Check sheet for the modelled part. Datum: model origin and axes. Units: mm. Face numbers are marked on the shaded views. A direction names the side the tool comes from. Round coordinates to 2 decimals unless told otherwise and drop trailing zeros. Loops run counter-clockwise (first coordinate to the right, second up) from the corner with the lowest first, then second, coordinate; pieces in that order, holes last. Notation, with made-up numbers: M 44,48 L 99,48 A19 cw 99,72 Z; hole C 15,-18 d11. An arc over 180 degrees is marked long. Write item = value, one per line. Start each with the question number.
(1) Cross-section at C-C on z = -1.25. Record the boundary of the cut face in (x, y), plus the area to 3 significant figures.
(2) Cross-section at B-B on x = -67.5. Record the boundary of the cut face in (y, z).
(3) Go/stop test with a flat-tipped pin: P1, Ø1, axis at x = -56, z = 2.5, coming from the -Y side. Record where the tip stops, or that it passes through.
(4) Scan lines: L1, parallel to Z at x = -48.5, y = 3; L2, parallel to Z at x = -27, y = -0.25; L3, parallel to X at y = -2, z = 0.75. Record each from-to range of solid material in increasing order. Write a range as from..to.
(5) Cross-section at A-A on y = 0. Record the boundary of the cut face in (x, z).
(6) Set-up check for the marked faces 1, 2 and 3: record each of +Z, -Z, +X, -X, +Y, -Y from which the full face is reachable in a straight line by a thin tool's end or side.
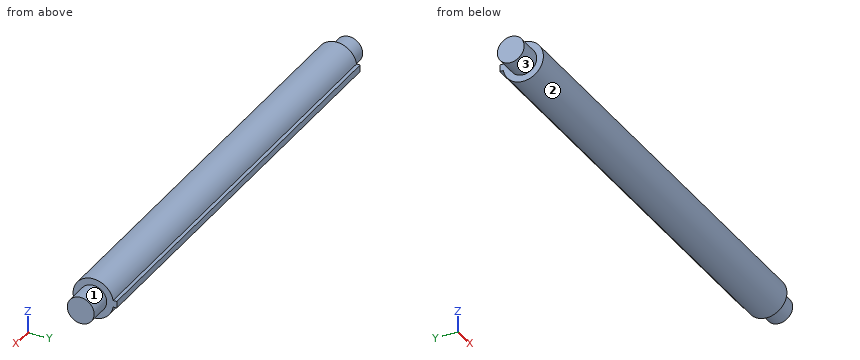
from build123d import *

# Parameters (mm, degrees)
SKETCH2_W           = 1
SKETCH2_H           = 1
BOSS_EXTRUDE1_DEPTH = 68


with BuildPart() as part:
    # Sketch1 → Revolve1 (revolve)
    with BuildSketch(Plane.XY):
        Polygon((0, 0), (-75, 0), (-75, 2), (-71.5, 2), (-71.5, 3), (-3.5, 3), (-3.5, 2), (0, 2), align=None)
    revolve(axis=Axis((0, 0, 0), (-1, 0, 0)))

    # Sketch2 → Boss-Extrude1 (add)
    with BuildSketch(Plane.ZY.offset(71.5)):
        with Locations((0, 3)):
            Rectangle(SKETCH2_W, SKETCH2_H)
    extrude(amount=-BOSS_EXTRUDE1_DEPTH)


solid = part.part
Result:
q1.outline = M -75,-1.56 L -71.5,-1.56 L -71.5,-2.73 L -3.5,-2.73 L -3.5,-1.56 L 0,-1.56 L 0,1.56 L -3.5,1.56 L -3.5,2.73 L -71.5,2.73 L -71.5,1.56 L -75,1.56 Z
q1.area = 393 mm^2
q2.outline = M 2.96,-0.5 L 3.5,-0.5 L 3.5,0.5 L 2.96,0.5 A3 ccw long Z
q3.P1 = -2.24
q4.L1 = -0.5..0.5
q4.L2 = -2.99..2.99
q4.L3 = -71.5..-3.5
q5.outline = M -75,-2 L -71.5,-2 L -71.5,-3 L -3.5,-3 L -3.5,-2 L 0,-2 L 0,2 L -3.5,2 L -3.5,3 L -71.5,3 L -71.5,2 L -75,2 Z
q6.face_1 = +X
q6.face_2 = +X, -X
q6.face_3 = -X
